Autodesk Inventor part; units mm, degrees
ref_plane "YZ Plane" through (0, 0, 0) normal (1, 0, 0) x (0, 1, 0)
ref_plane "XZ Plane" through (0, 0, 0) normal (0, 1, 0) x (-1, 0, 0)
ref_plane "XY Plane" through (0, 0, 0) normal (0, 0, 1) x (1, 0, 0)
sketch "草图1" plane through (0, 0, 0) normal (0, 1, 0) x (-1, 0, 0)
  line L0 (0, 0) -> (145, 0)
  line L1 (145, 0) -> (145, -65)
  line L2 (145, -65) -> (0, -65)
  line L3 (0, -65) -> (0, 0)
  dimension "d0" = 145
  dimension "d1" = 65
extrude "拉伸1" add sketch "草图1" along normal blind 2
sketch "草图2" plane through (0, 2, 0) normal (0, 1, 0) x (1, 0, 0)
  line L0 (-145, 0) -> (0, 0)
  line L1 (0, 0) -> (0, 2)
  line L2 (0, 0) -> (0, 65)
  line L3 (0, 2) -> (-12, 2)
  line L4 (-12, 2) -> (-12, 63)
  line L5 (-12, 2) -> (-89, 2)
  line L6 (-89, 2) -> (-89, 63)
  line L7 (-12, 2) -> (-12.9, 2)
  line L8 (-12.9, 2) -> (-12.9, 3)
  line L9 (-12.9, 3) -> (-11.1, 3)
  line L10 (-11.1, 3) -> (-11.1, 2)
  line L11 (-12, 63) -> (-12.9, 63)
  line L12 (-12.9, 63) -> (-12.9, 62)
  line L13 (-12.9, 62) -> (-11.1, 62)
  line L14 (-11.1, 62) -> (-11.1, 63)
  line L15 (-11.1, 63) -> (-12, 63)
  line L16 (-89, 63) -> (-88.1, 63)
  line L17 (-88.1, 63) -> (-88.1, 62)
  line L18 (-88.1, 62) -> (-89.9, 62)
  line L19 (-89.9, 62) -> (-89.9, 63)
  line L20 (-89.9, 63) -> (-88.1, 63)
  line L21 (-89, 2) -> (-89.9, 2)
  line L22 (-89.9, 2) -> (-89.9, 3)
  line L23 (-89.9, 3) -> (-88.1, 3)
  line L24 (-88.1, 3) -> (-88.1, 2)
  dimension "d4" = 2
  dimension "d5" = 12
  dimension "d6" = 61
  dimension "d7" = 77
  dimension "d8" = 0.9
  dimension "d9" = 1
  dimension "d10" = 1.8
  dimension "d11" = 1
  dimension "d12" = 0.9
  dimension "d13" = 1.8
extrude "拉伸2" add sketch "草图2" along normal blind 6
sketch "草图3" plane through (-89.9, 2, -3) normal (-1, 0, 0) x (0, 0, 1)
  line L0 (1, 0) -> (1, 6)
  line L1 (1, 6) -> (1, 4)
  line L2 (1, 4) -> (2, 4)
  line L3 (2, 4) -> (1, 6)
  line L4 (-60, 6) -> (-59, 6)
  line L5 (-60, 6) -> (-60, 4)
  line L6 (-60, 0) -> (-60, 6)
  line L7 (-60, 4) -> (-61, 4)
  line L8 (-61, 4) -> (-60, 6)
  point P0 (3, -2)
  dimension "d16" = 2
  dimension "d17" = 1
  dimension "d18" = 1
extrude "拉伸3" add sketch "草图3" against normal blind 1.8
sketch "草图4" plane through (-12.9, 2, -3) normal (-1, 0, 0) x (0, 0, 1)
  line L0 (1, 6) -> (2, 4)
  line L1 (2, 4) -> (1, 4)
  line L2 (1, 6) -> (2, 4)
  line L3 (2, 4) -> (1, 4)
  line L4 (1, 0) -> (1, 6)
  line L5 (1, 4) -> (1, 6)
  line L6 (-59, 6) -> (-60, 6)
  line L7 (-60, 6) -> (-60, 4)
  line L8 (-60, 0) -> (-60, 6)
  line L9 (-61, 4) -> (-60, 4)
  line L10 (-60, 6) -> (-61, 4)
  line L11 (-61, 4) -> (-60, 6)
  line L12 (-60, 0) -> (-60, 4)
  line L13 (-60, 6) -> (-60, 4)
  line L14 (-60, 4) -> (-61, 4)
  line L15 (1, 6) -> (0, 6)
  line L16 (1, 6) -> (1, 4)
  line L17 (1, 4) -> (2, 4)
  point P0 (3, -2)
extrude "拉伸4" add sketch "草图4" against normal blind 1.8
chamfer "倒角1" distance 0.5 angle 45 20 edges at (-72.5, 0, 0) (-145, 1, 0) (-145, 0, -32.5) (0, 1, 0) (-145, 1, -65) (-72.5, 0, -65) (0, 1, -65) (0, 0, -32.5) (-89, 2, -62) (-12, 2, -62) (-11.1, 2, -62.5) (-88.1, 2, -62.5) (-11.1, 2, -2.5) (-88.1, 2, -2.5) (-12.9, 2, -62.5) (-89.9, 2, -62.5) (-89.9, 2, -2.5) (-12.9, 2, -2.5) (-12, 2, -3) (-89, 2, -3)
sketch "草图5" plane through (0, 2, 0) normal (0, 1, 0) x (1, 0, 0)
  line L0 (-145, 64.5) -> (-145, 0.5)
  line L1 (-145, 64.5) -> (-143, 64.5)
  line L2 (-0.5, 64.5) -> (-144.5, 64.5)
  line L3 (-0.5, 65) -> (-144.5, 65)
  line L4 (-143, 65) -> (-115, 65)
  line L5 (-143, 65) -> (-143, 37)
  line L6 (-143, 37) -> (-143, 29)
  line L7 (-143, 37) -> (-141, 37)
  line L8 (-141, 37) -> (-141, 29)
  line L9 (-141, 29) -> (-143, 29)
  point P0 (0, 0)
  dimension "d26" = 2
  dimension "d27" = 28
  dimension "d28" = 28
  dimension "d29" = 8
  dimension "d30" = 2
extrude "拉伸5" add sketch "草图5" along normal blind 4
sketch "草图6" plane through (-143, 2, -29) normal (0, 0, 1) x (1, 0, 0)
  line L0 (0, 4) -> (2, 4)
  line L1 (0, 4) -> (0, 2)
  line L2 (0, 0) -> (0, 4)
  line L3 (0, 2) -> (-1, 2)
  line L4 (-1, 2) -> (0, 4)
  point P0 (143, -2)
  dimension "d33" = 2
  dimension "d34" = 1
extrude "拉伸6" add sketch "草图6" against normal blind 8
chamfer "倒角2" distance 0.5 angle 45 3 edges at (-141, 2, -33) (-142, 2, -29) (-142, 2, -37)
sketch "草图7" plane through (0, 2, 0) normal (0, 1, 0) x (1, 0, 0)
  line L0 (-144.5, 65) -> (-145, 64.5)
  line L1 (-145, 64.5) -> (-140.3, 64.5)
  line L2 (-0.5, 64.5) -> (-144.5, 64.5)
  line L3 (-140.3, 64.5) -> (-140.3, 65)
  line L4 (-0.5, 65) -> (-144.5, 65)
  line L5 (-140.3, 65) -> (-140.3, 60.3)
  line L6 (-140.3, 60.3) -> (-140.3, 5.6)
  line L7 (-140.3, 5.6) -> (-115.535, 5.6)
  line L8 (-115.535, 5.6) -> (-115.535, 60.3)
  line L9 (-115.535, 60.3) -> (-140.3, 60.3)
  circle A0 centre (-140.3, 60.3) radius 1.6
  circle A1 centre (-140.3, 60.3) radius 2.5
  circle A2 centre (-115.535, 60.3) radius 1.6
  circle A3 centre (-115.535, 60.3) radius 2.5
  circle A4 centre (-115.535, 5.6) radius 1.6
  circle A5 centre (-115.535, 5.6) radius 2.5
  circle A6 centre (-140.3, 5.6) radius 1.6
  circle A7 centre (-140.3, 5.6) radius 2.5
  point P0 (0, 0)
  dimension "d40" = 4.7
  dimension "d41" = 4.7
  dimension "d44" = 54.7
  dimension "d45" = 24.765
  dimension "d46" = 3.2
  dimension "d47" = 5
  dimension "d48" = 3.2
  dimension "d49" = 5
  dimension "d50" = 3.2
  dimension "d51" = 5
  dimension "d52" = 3.2
  dimension "d53" = 5
extrude "拉伸7" add sketch "草图7" along normal blind 5 contours A1 L9 A0 L5 | L5 A0 L6 A1 | A1 L6 A0 L9 | A3 L8 A2 L9 | L9 A2 L8 A3 | A7 L7 A6 L6 | L6 A6 L7 A7 | A5 L7 A4 L8 | L8 A4 L7 A5
chamfer "倒角3" distance 0.5 angle 45 13 edges at (-142.8, 2, -60.3) (-118.035, 2, -60.3) (-142.8, 2, -5.6) (-118.035, 2, -5.6) (-141.9, 7, -5.6) (-117.135, 7, -5.6) (-141.9, 7, -60.3) (-117.135, 7, -60.3) (-141, 6, -33) (-89, 8, -62) (-12, 8, -62) (-12, 8, -3) (-89, 8, -3)
properties part number "BOT" material "酚醛树脂"
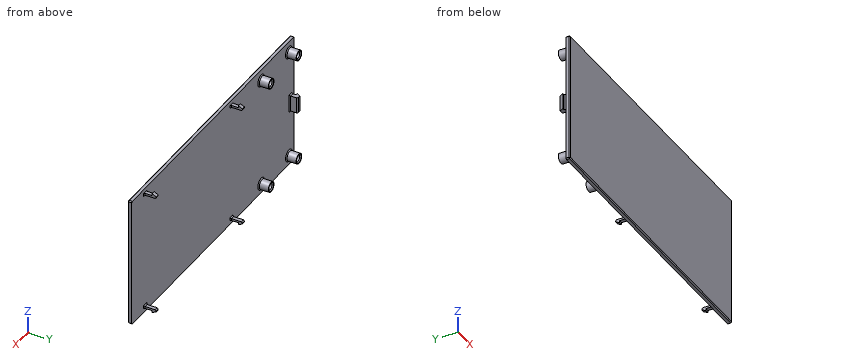
Input: part model. Units: mm. Frame: model coordinates. Coordinates: 2 decimals unless noted, no trailing zeros. Write each loop counter-clockwise with the first axis right and the second up, starting at its lowest first coordinate (ties: lowest second). Pieces come first, ordered by that corner, then holes. Notation, with made-up numbers: (66, 50.25) -> (102, 50.25) arc R18 cw to (102, 61.25) -> close; hole circle Ø9 at (33, 77). An arc over 180 degrees is marked (long way). Write each question's results on one line, items separated by ' | '.
Item 1: Section query B-B on x = -98. Return loops of the section in (y, z).
Conclusion:
outline: (0, -64.5) -> (0.5, -65) -> (2, -65) -> (2, 0) -> (0.5, 0) -> (0, -0.5) -> close
Item 2: Pin query (flat end, axial travel): pin 1 Ø5 at (x, z) = (-72.5, -51.5) entering from +Y; pin 2 Ø2 at (x, y) = (-89.5, 4.5) entering from +Z; pin 3 Ø1 at (y, z) = (5.5, -63) entering from -X; pin 4 Ø1.5 at (x, y) = (-102, 3) entering from +Z. Return the tip coordinate at first contact, or that it passes through.
Conclusion:
pin 1: stops at y = 2 | pin 2: stops at z = -2 | pin 3: stops at x = -141.49 | pin 4: passes through
Item 3: Material intervals for probe 1 along X at (y, z) = (3.6, -60.3) (3 decimals); probe 2 along Z at (x, y) = (-140.3, 3.2); probe 3 along Y at (x, z) = (-9.5, -50), sorted ascending.
Conclusion:
probe 1: x = -142.8 to -141.9, -138.7 to -137.8, -118.035 to -117.135, -113.935 to -113.035 | probe 2: z = -62.8 to -61.9, -58.7 to -57.8, -8.1 to -7.2, -4 to -3.1 | probe 3: y = 0 to 2
Item 4: Section query C-C on z = -54.5. Return loops of the section in (x, y), plus the area to 3 significant figures.
Conclusion:
outline: (-145, 0.5) -> (-144.5, 0) -> (-0.5, 0) -> (0, 0.5) -> (0, 2) -> (-145, 2) -> close | area: 290 mm^2
